Autodesk Inventor part; units mm, degrees
ref_plane "YZ Plane" through (0, 0, 0) normal (1, 0, 0) x (0, 1, 0)
ref_plane "XZ Plane" through (0, 0, 0) normal (0, 1, 0) x (-1, 0, 0)
ref_plane "XY Plane" through (0, 0, 0) normal (0, 0, 1) x (1, 0, 0)
sketch "Sketch1" plane through (0, 0, 0) normal (0, 0, 1) x (1, 0, 0)
  circle A0 centre (0, 0) radius 35
  line L0 (0, 35) -> (212.4975, 35)
  line L1 (212.4975, 35) -> (294.7487, -47.2513)
  circle A1 centre (270, -72) radius 35
  line L2 (0, -35) -> (183.5025, -35)
  line L3 (183.5025, -35) -> (245.2513, -96.7487)
  dimension "d0" = 70
  dimension "d1" = 135
  dimension "d2" = 70
  dimension "d3" = 37
  dimension "d4" = 270
extrude "Extrusion1" add sketch "Sketch1" along normal blind 22.5
sketch "Sketch2" plane through (0, 0, 22.5) normal (0, 0, 1) x (1, 0, 0)
  line L0 (294.7487, -47.2513) -> (212.4975, 35)
  line L1 (212.4975, 35) -> (142.4975, -35)
  line L2 (0, -35) -> (183.5025, -35)
  arc A0 (245.2513, -96.7487) -> (294.7487, -47.2513) centre (270, -72) ccw
  line L3 (294.7487, -47.2513) -> (212.4975, 35)
  line L4 (212.4975, 35) -> (0, 35)
  arc A1 (0, 35) -> (0, -35) centre (0, 0) ccw
  line L5 (0, -35) -> (183.5025, -35)
  line L6 (183.5025, -35) -> (245.2513, -96.7487)
  line L7 (142.4975, -35) -> (183.5025, -35)
  dimension "d7" = 45
extrude "Extrusion2" add sketch "Sketch2" along normal blind 12.5 contours A0 L6 L2 L1 L0
chamfer "Chamfer1" distance 12.5 angle 45 1 edges at (177.4975, 0, 22.5)
sketch "Sketch3" plane through (0, 0, 0) normal (0, 0, -1) x (-1, 0, 0)
  line L0 (-29, 10) -> (11, 10)
  line L1 (11, 10) -> (11, -10)
  line L2 (11, -10) -> (-29, -10)
  line L3 (-29, -10) -> (-29, 10)
  line L4 (11, 7) -> (21, 7)
  line L5 (21, 7) -> (21, -7)
  line L6 (21, -7) -> (11, -7)
  line L7 (11, -7) -> (11, 7)
  line L8 (21, 7) -> (21, 10)
  line L9 (21, 10) -> (3.9289, 27.0711)
  line L10 (16.9289, 7) -> (3.9289, 20)
  line L11 (-212.4975, 35) -> (0, 35)
  line L12 (3.9289, 20) -> (3.9289, 27.0711) construction
  line L13 (3.9289, 27.0711) -> (-204.5685, 27.0711)
  line L14 (3.9289, 20) -> (-197.4975, 20)
  line L15 (-212.4975, 35) -> (-142.4975, -35) construction
  line L16 (-204.5685, 27.0711) -> (-264.6396, -33)
  line L17 (-204.5685, 27.0711) -> (-130.9289, 27.0711) construction
  line L18 (-197.4975, 20) -> (-250.4975, -33)
  line L19 (-294.7487, -47.2513) -> (-212.4975, 35)
  line L20 (0, -35) -> (-183.5025, -35)
  line L21 (-264.6396, -33) -> (-250.4975, -33)
  point P0 (0, 0)
  point P1 (-194.8198, 35)
  dimension "d13" = 40
  dimension "d14" = 20
  dimension "d15" = 10
  dimension "d16" = 29
  dimension "d17" = 3
  dimension "d18" = 3
  dimension "d19" = 10
  dimension "d22" = 135
  dimension "d23" = 3
  dimension "d24" = 10
  dimension "d25" = 5
  dimension "d26" = 10
  dimension "d29" = 135
  dimension "d35" = 2
sketch "Sketch4" plane through (0, 0, 0) normal (0, 0, -1) x (-1, 0, 0)
  line L0 (-142.4975, -35) -> (-183.5025, -35)
  line L1 (-183.5025, -35) -> (-282.4975, -35)
  line L2 (-294.7487, -47.2513) -> (-212.4975, 35)
  line L3 (0, -35) -> (-183.5025, -35)
  arc A0 (-294.7487, -47.2513) -> (-245.2513, -96.7487) centre (-270, -72) ccw
  line L4 (-183.5025, -35) -> (-245.2513, -96.7487)
  line L5 (0, -35) -> (-183.5025, -35)
  arc A1 (0, -35) -> (0, 35) centre (0, 0) ccw
  line L6 (-212.4975, 35) -> (0, 35)
  line L7 (-294.7487, -47.2513) -> (-212.4975, 35)
  line L8 (-282.4975, -35) -> (-294.7487, -47.2513)
extrude "Extrusion3" cut sketch "Sketch4" against normal blind 22.5 contours L4 A0 L2 L1
extrude "Extrusion4" cut sketch "Sketch3" against normal blind 20
sketch "Sketch5" plane through (0, 0, 22.5) normal (0, 0, 1) x (1, 0, 0)
  circle A0 centre (0, 0) radius 12.5
  dimension "d30" = 25
extrude "Extrusion5" add sketch "Sketch5" along normal blind 5
sketch "Sketch6" plane through (0, 0, 20) normal (0, 0, -1) x (-1, 0, 0)
  line L0 (11, 7) -> (16.9289, 7)
  line L1 (11, 10) -> (11, 7)
  line L2 (-29, 10) -> (11, 10)
  line L3 (-29, -10) -> (-29, 10)
  line L4 (11, -10) -> (-29, -10)
  line L5 (11, -7) -> (11, -10)
  line L6 (21, -7) -> (11, -7)
  line L7 (21, 10) -> (21, -7)
  line L8 (3.9289, 27.0711) -> (21, 10)
  line L9 (-204.5685, 27.0711) -> (3.9289, 27.0711)
  line L10 (-264.6396, -33) -> (-204.5685, 27.0711)
  line L11 (-250.4975, -33) -> (-264.6396, -33)
  line L12 (-197.4975, 20) -> (-250.4975, -33)
  line L13 (3.9289, 20) -> (-197.4975, 20)
  line L14 (16.9289, 7) -> (3.9289, 20)
  line L15 (-264.6396, -33) -> (-204.5685, 27.0711)
  line L16 (-254.6396, -23) -> (-240.4975, -23)
  line L17 (-197.4975, 20) -> (-250.4975, -33)
  point P0 (0, 0)
  dimension "d36" = 10
extrude "Extrusion6" cut sketch "Sketch6" against normal up to surface (2.5 mm away) contours L12 L11 L10 L16
sketch "Sketch7" plane through (0, 0, 22.5) normal (0, 0, -1) x (-1, 0, 0)
  line L0 (-254.6396, -23) -> (-240.4975, -23)
  line L1 (-264.6396, -33) -> (-254.6396, -23)
  line L2 (-250.4975, -33) -> (-264.6396, -33)
  line L3 (-240.4975, -23) -> (-250.4975, -33)
  line L4 (-264.6396, -33) -> (-280, -48.3604)
  line L5 (-280, -48.3604) -> (-265.8579, -48.3604)
  line L6 (-265.8579, -48.3604) -> (-250.4975, -33)
  point P0 (0, 0)
extrude "Extrusion7" cut sketch "Sketch7" against normal blind 10
sketch "Sketch8" plane through (0, 0, 22.5) normal (0, 0, -1) x (-1, 0, 0)
  arc A0 (-294.7487, -47.2513) -> (-245.2513, -96.7487) centre (-270, -72) ccw
  circle A1 centre (-270, -72) radius 12.5
  point P0 (0, 0)
  dimension "d41" = 25
extrude "Extrusion8" cut sketch "Sketch8" against normal blind 5
properties part number "arm 1 leftt"
Source: CAD feature listing. Evaluate the final solid. Frame: model axes, mm. A direction names the side the tool comes from. Coordinates: 2 decimals unless noted, no trailing zeros. Loops run counter-clockwise (first coordinate to the right, second up) from the corner with the lowest first, then second, coordinate; pieces in that order, holes last. Notation, with made-up numbers: (0, 22.5) - (31, 22.5) arc R15 cw to (31, 30.5) - close; hole circle Ø10 at (30.25, 76). An arc over 180 degrees is marked (long way). One line per item, written item: value. Start each with the question number.
1. Set-up query: faces 4 (the flat face through (254.2, -6.7, 17.3)), 5 (the cylindrical face through (11.923, -3.755, 24.965)), 6 (the flat face through (0, 0, 27.5)), 7 (the flat face through (29, 0, 10)). Return all of +Z, -Z, +X, -X, +Y, -Y with unobstructed straight access to the full face (end or side cutting, diameter ignored); none if empty.
2. Mould query, pull axis Y, two halves, no side actions, for faces 1 (the flat face through (259, -62, 22.5)), 2 (the cylindrical face through (258.077, -68.245, 24.965)), 3 (the flat face through (213.9, -65.4, 28.7)). Classes: pulls with the +Y half, pulls with the -Y half, needs draft (parallel to the pull), parting line crosses it, or undercut.
3. Contact query for flat-ended pins moving along their axis: P1, Ø3, axis at x = -13.5, z = 6.5, coming from the -Y side; P2, Ø1.5, axis at y = 8, z = 14, coming from the +X side; P3, Ø12, axis at x = 40, z = 16.5, coming from the -Y side. Output: stop coordinate, or through.
4. Section C-C (y = -76). Return the cut outline in (x, z).
5. Ray query, L1, parallel to Y at x = 16, z = 1.5; L2, parallel to Y at x = 270, z = 25.45; L3, parallel to X at y = 6, z = 16.5. Return the intervals inside material, ascending.
6. Section A-A (x = 80). Return the cut outline in (y, z), and give its area (3 significant figures).
7. Section D-D (x = 274). Return the cut outline in (y, z).
8. Section B-B (z = 4.5). Return the cut outline in (x, y).
Verdict:
1. face 4: +Z, -Z, +X, +Y
1. face 5: +Z
1. face 6: +Z, -X, +Y, -Y
1. face 7: -Z
2. face 1: needs draft
2. face 2: undercut
2. face 3: pulls with the -Y half
3. P1: stops at y = -32.88
3. P2: stops at x = 240.25
3. P3: stops at y = -35
4. outline: (224.5, 22.5) - (258.16, 22.5) - (258.16, 27.5) - (281.84, 27.5) - (281.84, 22.5) - (304.77, 22.5) - (304.77, 35) - (224.5, 35) - close
5. L1: y = -35 to -10, 10 to 20, 27.07 to 35
5. L2: y = -107 to -84.5, -59.5 to -48.36, -38.36 to -22.5
5. L3: x = -34.48 to -21, 29 to 211.5, 225.64 to 241.5
6. outline: (-35, 0) - (20, 0) - (20, 20) - (27.07, 20) - (27.07, 0) - (35, 0) - (35, 22.5) - (-35, 22.5) - close
6. area: 1,430 mm2
7. outline: (-106.77, 22.5) - (-83.84, 22.5) - (-83.84, 27.5) - (-60.16, 27.5) - (-60.16, 22.5) - (-48.36, 22.5) - (-48.36, 32.5) - (-42.36, 32.5) - (-42.36, 22.5) - (-35, 22.5) - (-35, 0) - (-26.5, 0) - (-26.5, 35) - (-106.77, 35) - close
8. outline: (0, -35) - (282.5, -35) - (212.5, 35) - (0, 35) arc R35 ccw to start; hole (-21, -7) - (-11, -7) - (-11, -10) - (29, -10) - (29, 10) - (-11, 10) - (-11, 7) - (-16.93, 7) - (-3.93, 20) - (197.5, 20) - (250.5, -33) - (264.64, -33) - (204.57, 27.07) - (-3.93, 27.07) - (-21, 10) - close
